Autodesk Inventor part; units mm, degrees
ref_plane "IP1_XY" through (0, 0, 0) normal (1, 0, 0) x (0, 0, -1)
ref_plane "IP1_YZ" through (0, 0, 0) normal (0, 0, -1) x (0, 1, 0)
ref_plane "IP1_ZX" through (0, 0, 0) normal (0, 1, 0) x (1, 0, 0)
sketch "Skizze_2" plane through (0, 0, 0) normal (0, 0, 1) x (1, 0, 0)
  line L0 (20, 0) -> (-0.7453, 0)
  line L1 (-0.7453, 0) -> (-1.9, 2)
  line L2 (-1.9, 2) -> (-5, 2)
  line L3 (-5, 2) -> (-5, 3.75)
  arc A0 (-4.5, 4.25) -> (-5, 3.75) centre (-4.5, 3.75) ccw
  line L4 (-4.5, 4.25) -> (0, 4.25)
  line L5 (0, 4.25) -> (0, 2.85)
  arc A1 (0, 2.85) -> (0.1298, 2.6627) centre (0.2, 2.85) ccw
  line L6 (0.1298, 2.6627) -> (0.5298, 2.5127)
  arc A2 (0.5298, 2.5127) -> (0.6, 2.5) centre (0.6, 2.7) ccw
  line L7 (0.6, 2.5) -> (19.5095, 2.5)
  line L8 (19.5095, 2.5) -> (20, 2.0095)
  line L9 (20, 2.0095) -> (20, 0)
  line L10 (20, 0) -> (-0.7453, 0)
revolve "Revolution1" add sketch "Skizze_2" angle 360 about axis through (20, 0, 0) along (1, 0, 0)
thread "Thread1"
sketch "Skizze_1" plane through (-1.9, 0, 0) normal (1, 0, 0) x (0, 0, -1)
  line L0 (-2, 1.1547) -> (-2, -1.1547)
  line L1 (-2, -1.1547) -> (0, -2.3094)
  line L2 (0, -2.3094) -> (2, -1.1547)
  line L3 (2, -1.1547) -> (2, 1.1547)
  line L4 (2, 1.1547) -> (0, 2.3094)
  line L5 (0, 2.3094) -> (-2, 1.1547)
extrude "Extrusion1" cut sketch "Skizze_1" against normal blind 5
ref_plane "IP1_XY" through (0, 0, 0) normal (1, 0, 0) x (0, 0, -1)
ref_plane "IP1_YZ" through (0, 0, 0) normal (0, 0, -1) x (0, 1, 0)
ref_plane "IP1_ZX" through (0, 0, 0) normal (0, 1, 0) x (1, 0, 0)
ref_plane "IP2_XY" through (-5, 0, 0) normal (1, 0, 0) x (0, 0, -1)
ref_plane "IP2_YZ" through (-5, 0, 0) normal (0, 0, -1) x (0, 1, 0)
ref_plane "IP2_ZX" through (-5, 0, 0) normal (0, 1, 0) x (1, 0, 0)
ref_plane "IP3_XY" through (20, 0, 0) normal (1, 0, 0) x (0, 0, -1)
ref_plane "IP3_YZ" through (20, 0, 0) normal (0, 0, -1) x (0, 1, 0)
ref_plane "IP3_ZX" through (20, 0, 0) normal (0, 1, 0) x (1, 0, 0)
ref_plane "IP4_XY" through (0, 0, 0) normal (1, 0, 0) x (0, 0, -1)
ref_plane "IP4_YZ" through (0, 0, 0) normal (0, 0, -1) x (0, 1, 0)
ref_plane "IP4_ZX" through (0, 0, 0) normal (0, 1, 0) x (1, 0, 0)
properties part number "Slotted head cap screw ISO 4762 - M5x20"
Here's how the part is built. I have some questions about the finished solid (model axes, mm). A direction names the side the tool comes from. Give positions to 0.01 mm unless a question says otherwise; leave off trailing zeros. Order: outer loops, then holes, each group sorted by start corner. A loop starts at its lowest first (then second) coordinate and runs counter-clockwise, first axis right, second up. Notation, with made-up numbers: (19.25, 81.5) - (39.25, 81.5) arc R18 cw to (39.25, 114.5) - close; hole circle Ø9 at (82, 60). An arc over 180 degrees is marked (long way). Answer as a JSON object with one key per item and string values. Group by question number.
Item 1: Please list where these lines run through material, in increasing order: probe 1 along X at (y, z) = (0.75, 3); probe 2 along Y at (x, z) = (-0.5, 2); probe 3 along Y at (x, z) = (0.25, -0.25).
Item 2: If we section it at A-A on x = 5.75: Please give me the cut outline in (y, z), and give its area (3 significant figures).
Item 3: Which directions (+Z, -Z, +X, -X, +Y, -Y) give clear straight access to the entire face, cutting with the end or side of a thin tool? Please do faces 1 (the flat face through (-3.428, -1.724, 1.014)), 2 (the flat face through (0, 1, -3)), 3 (the flat face through (-5, 2, -2)).
Item 4: For P1, Ø5, axis at y = -2.5, z = 0, coming from the +X side; P2, Ø4, axis at x = 10, z = -2, coming from the -Y side; P3, Ø5, axis at x = 6, z = -0.5, coming from the +Y side; P4, Ø2, axis at x = 16.5, z = 2.5, coming from the +Y side, each with a flat end and sliding along its axis, tell me the tip position at first contact or that it passes through.
Item 5: If we mould it in two halves opening along Y, with no side actions, what happens to faces 4 (the conical face through (-0.946, -0.256, -0.235)), 5 (the cylindrical face through (-2.218, 2.285, 3.584)), 6 (the flat face through (20, 0, 0))? For each: pulls with the +Y half, pulls with the -Y half, needs draft (parallel to the pull), parting line crosses it, or undercut.
Result set:
{
 "1": {"probe 1": "-5 to 0", "probe 2": "-3.75 to 3.75", "probe 3": "-2.61 to 2.61"},
 "2": {"outline": "circle Ø5 at (0, 0)", "area": "19.6 mm²"},
 "3": {"face 1": "-X", "face 2": "+X", "face 3": "+Z, -Z, -X, +Y, -Y"},
 "4": {"P1": "x = 20", "P2": "y = -2.5", "P3": "y = 2.5", "P4": "y = 2"},
 "5": {"face 4": "undercut", "face 5": "parting line crosses it", "face 6": "needs draft"}
}
